Here's how the part is built. I have some questions about the finished solid (model axes, mm). A direction names the side the tool comes from. Give positions to 0.01 mm unless a question says otherwise; leave off trailing zeros. Order: outer loops, then holes, each group sorted by start corner. A loop starts at its lowest first (then second) coordinate and runs counter-clockwise, first axis right, second up.
from build123d import *

# Parameters (mm, degrees)
SKETCH1_W           = 38.1
SKETCH1_H           = 19.05
BOSS_EXTRUDE1_DEPTH = 304.8
CUT_EXTRUDE1_REACH  = 309.762
SKETCH2_W           = 25.4
SKETCH2_H           = 12.7


with BuildPart() as part:
    # Sketch1 → Boss-Extrude1 (new body)
    with BuildSketch(Plane.XY):
        with Locations((19.05, 9.525)):
            Rectangle(SKETCH1_W, SKETCH1_H)
    extrude(amount=BOSS_EXTRUDE1_DEPTH)

    # Sketch2 → Cut-Extrude1 (cut, up to next)
    with BuildSketch(Plane.XY.offset(304.8), mode=Mode.PRIVATE) as cut_extrude1_sk1:
        with Locations((19.05, 12.7)):
            Rectangle(SKETCH2_W, SKETCH2_H)
    cut_extrude1_tool1 = extrude(cut_extrude1_sk1.sketch, amount=-CUT_EXTRUDE1_REACH, mode=Mode.PRIVATE) & part.part
    add(cut_extrude1_tool1.solids().sort_by_distance((19.05, 12.7, 304.8))[0], mode=Mode.SUBTRACT)


solid = part.part
Q1. Thinking about a two-plate mould opening in X: for faces 3 (the face through (3, 19.05, 150)), 4 (the face through (38.1, 9, 150)), 5 (the face through (6.35, 13, 155)), 6 (the face through (0, 9, 150)), which applies, released by +X, released by -X, zero draft, split by the parting line, or undercut?
Filled sheet:
face 3: zero draft
face 4: released by +X
face 5: undercut
face 6: released by -X
Q2. For faces 1 (the face through (19, 0, 150)), 2 (the face through (31.75, 13, 155)), which set-ups out of +Z, -Z, +X, -X, +Y, -Y let a thin tool reach every point of the face, with its end or its side?
Filled sheet:
face 1: +Z, -Z, +X, -X, -Y
face 2: +Z, -Z, +Y
Q3. I'm going to push a flat-ended pin straight in: P1, Ø12.5, axis at x = 15.5, z = 182.5, coming from the +Y side. Where does the tip first touch, or does it pass through?
Filled sheet:
P1: stops at y = 6.35
Q4. I need wall thicknesses on L1, parallel to X at y = 14, z = 260; L2, parallel to Y at x = 30, z = 94.5. Which ranges of each line are inside material? Lowest first, please.
Filled sheet:
L1: x = 0 to 6.35, 31.75 to 38.1
L2: y = 0 to 6.35
Q5. If we section it at C-C on x = 10: List the corners of the cut face in (y, z) for me.
Filled sheet:
outline: (0, 0) - (6.35, 0) - (6.35, 304.8) - (0, 304.8) - close
Q6. If we section it at A-A on y = 14.5: List the corners of the cut face in (x, z) for me.
Filled sheet:
outline: (0, 0) - (6.35, 0) - (6.35, 304.8) - (0, 304.8) - close; (31.75, 0) - (38.1, 0) - (38.1, 304.8) - (31.75, 304.8) - close
Q7. If we section it at B-B on z = 175: List the corners of the cut face in (x, y) for me, plus the area to 3 significant figures.
Filled sheet:
outline: (0, 0) - (38.1, 0) - (38.1, 19.05) - (31.75, 19.05) - (31.75, 6.35) - (6.35, 6.35) - (6.35, 19.05) - (0, 19.05) - close
area: 403 mm2
